Work out the finished part from the listing and answer in its coordinate system (mm). Face numbers are marked on the shaded views. Coordinates: 2 decimals unless noted, no trailing zeros. Loops run counter-clockwise (first coordinate to the right, second up) from the corner with the lowest first, then second, coordinate; pieces in that order, holes last.
```python
from build123d import *

# Parameters (mm, degrees)
SKETCH1_W                 = 146.7
SKETCH1_H                 = 71.5
BASE_DEPTH                = 7.65
CURVES_CASE_R             = 5
SHELL_T                   = -1.5
CAMERA_HOLE_DEPTH         = 82.956131558
CAMERA_HOLE_DEPTH_BACK    = 82.956131558
SKETCH2_W                 = 25
SKETCH2_H                 = 25
CURVES_CAMERA_R           = 5
CHARGER_BOTTOM_DEPTH      = 152.186887659
CHARGER_BOTTOM_DEPTH_BACK = 9.65
VOLUME_BOTTOM_DEPTH       = 0.65
TURN_ON_OFF_DEPTH         = 0.65


with BuildPart() as part:
    # Sketch1 → Base (new body)
    with BuildSketch(Plane(origin=(0, 0, 0), x_dir=(1, 0, 0), z_dir=(0, 1, 0))):
        Rectangle(SKETCH1_W, SKETCH1_H)
    extrude(amount=BASE_DEPTH)

    # Curves case
    curves_case_edges = [part.edges().sort_by_distance(p)[0] for p in [
        (73.35, 3.825, 35.75),
        (-73.35, 3.825, 35.75),
        (-73.35, 3.825, -35.75),
        (73.35, 3.825, -35.75),
    ]]
    fillet(curves_case_edges, radius=CURVES_CASE_R)

    # Shell
    shell_openings = [part.faces().sort_by_distance(p)[0] for p in [
        (0, 0, 0),
    ]]
    offset(amount=SHELL_T, openings=shell_openings, kind=Kind.INTERSECTION)

    # Sketch2 → Camera Hole (cut, two sides: drawn at the far end of the back side and taken through both)
    with BuildSketch(Plane(origin=(0, 7.65, 0), x_dir=(1, 0, 0), z_dir=(0, 1, 0)).offset(-CAMERA_HOLE_DEPTH_BACK)):
        with Locations((56.945704346, 19.35)):
            Rectangle(SKETCH2_W, SKETCH2_H)
    extrude(amount=CAMERA_HOLE_DEPTH + CAMERA_HOLE_DEPTH_BACK, mode=Mode.SUBTRACT)

    # Curves Camera
    curves_camera_edges = [part.edges().sort_by_distance(p)[0] for p in [
        (69.445704346, 6.9, -31.85),
        (69.445704346, 6.9, -6.85),
        (44.445704346, 6.9, -6.85),
        (44.445704346, 6.9, -31.85),
    ]]
    fillet(curves_camera_edges, radius=CURVES_CAMERA_R)

    # Sketch6 → Charger bottom (cut, two sides: drawn at the far end of the back side and taken through both)
    with BuildSketch(Plane.ZY.offset(73.35).offset(-CHARGER_BOTTOM_DEPTH_BACK)):
        with BuildLine():
            Line((-2.425, 4.722712559), (2.425, 4.722712559))
            ThreePointArc((2.425, 4.722712559), (4.087430665, 3.060281894), (2.425, 1.397851228))
            Line((2.425, 1.397851228), (-2.425, 1.397851228))
            ThreePointArc((-2.425, 1.397851228), (-4.087430665, 3.060281894), (-2.425, 4.722712559))
        make_face()
    extrude(amount=CHARGER_BOTTOM_DEPTH + CHARGER_BOTTOM_DEPTH_BACK, mode=Mode.SUBTRACT)

    # Sketch9 → Volume Bottom (add)
    with BuildSketch(Plane.XY.offset(35.75)):
        with BuildLine():
            Line((5.40710355, 5.075), (15.40710355, 5.075))
            ThreePointArc((15.40710355, 5.075), (16.65710355, 3.825), (15.40710355, 2.575))
            Line((15.40710355, 2.575), (5.40710355, 2.575))
            ThreePointArc((5.40710355, 2.575), (4.15710355, 3.825), (5.40710355, 5.075))
        make_face()
        with BuildLine():
            Line((18.803853298, 5.075), (28.803853298, 5.075))
            ThreePointArc((28.803853298, 5.075), (30.053853298, 3.825), (28.803853298, 2.575))
            Line((28.803853298, 2.575), (18.803853298, 2.575))
            ThreePointArc((18.803853298, 2.575), (17.553853298, 3.825), (18.803853298, 5.075))
        make_face()
    extrude(amount=VOLUME_BOTTOM_DEPTH)

    # Sketch11 → Turn on/off (add)
    with BuildSketch(Plane(origin=(0, 0, -35.75), x_dir=(-1, 0, 0), z_dir=(0, 0, -1))):
        with BuildLine():
            Line((-20.994631551, 5.075), (-6.504836948, 5.075))
            ThreePointArc((-6.504836948, 5.075), (-5.254836948, 3.825), (-6.504836948, 2.575))
            Line((-6.504836948, 2.575), (-20.994631551, 2.575))
            ThreePointArc((-20.994631551, 2.575), (-22.244631551, 3.825), (-20.994631551, 5.075))
        make_face()
    extrude(amount=TURN_ON_OFF_DEPTH)


solid = part.part
```
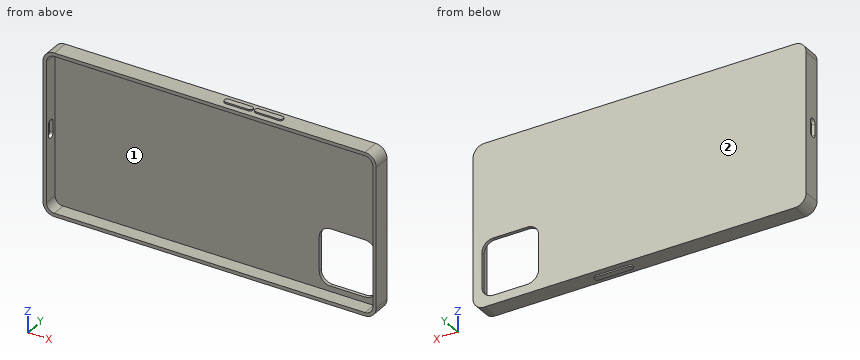
1. Determine the mould class of the marked faces 1 and 2 for opening direction Z: released by +Z, released by -Z, zero draft, split by the parting line, or undercut.
2. A cutting plane is placed at A-A, the plane z = -15. Give the vertices of the cut face in (x, y), then the cut area to 3 significant figures.
3. A cutting plane is placed at C-C, the plane z = 10.5. Give the vertices of the cut face in (x, y), then the cut area to 4 significant figures.
4. Straight lines are drawn through the part: probe 1 along X at (y, z) = (3.5, -29.5); probe 2 along Z at (x, y) = (-62, 1.5); probe 3 along Z at (x, y) = (5.5, 5). For each, find the intervals that lie inside material, in ascending order.
5. Each of these flat-tipped pins is pushed along its axis until it touches: P1, Ø1.2, axis at x = 57.5, y = 7, coming from the -Z side; P2, Ø10, axis at x = 42.5, z = -25, coming from the -Y side. Where does it stop, or does it pass through?
6. A cutting plane is placed at B-B, the plane x = -54. Give the vertices of the cut face in (y, z), then the cut area to 3 significant figures.
Answers below:
1. face 1: undercut
1. face 2: zero draft
2. outline: (-73.35, 0) - (-71.85, 0) - (-71.85, 6.15) - (44.45, 6.15) - (44.45, 7.65) - (-73.35, 7.65) - close; (69.45, 6.15) - (71.85, 6.15) - (71.85, 0) - (73.35, 0) - (73.35, 7.65) - (69.45, 7.65) - close
2. area: 201 mm2
3. outline: (-73.35, 0) - (-71.85, 0) - (-71.85, 6.15) - (71.85, 6.15) - (71.85, 0) - (73.35, 0) - (73.35, 7.65) - (-73.35, 7.65) - close
3. area: 238.5 mm2
4. probe 1: x = -73.35 to -71.85, 71.85 to 73.35
4. probe 2: z = -35.75 to -34.25, 34.25 to 35.75
4. probe 3: z = -35.75 to -34.25, 34.25 to 36.4
5. P1: stops at z = -35.75
5. P2: stops at y = 6.15
6. outline: (0, -35.75) - (7.65, -35.75) - (7.65, 35.75) - (0, 35.75) - (0, 34.25) - (6.15, 34.25) - (6.15, -34.25) - (0, -34.25) - close
6. area: 126 mm2
